Geometry: final body of the model. Coordinates: model frame, mm. A direction names the side the tool comes from. Give positions to 0.01 mm unless a question says otherwise; leave off trailing zeros. Write each loop counter-clockwise with the first axis right and the second up, starting at its lowest first coordinate (ties: lowest second). Pieces come first, ordered by that corner, then holes. Notation, with made-up numbers: M 47.25,86.25 L 96.25,86.25 A5 ccw 96.25,92.25 Z; hole C 36.5,42 d8. An arc over 180 degrees is marked long. Use one line per item in the form item = value. Start each with the question number.
Item 1: Section query D-D on x = -6.5. Return loops of the section in (y, z), then the cut area to 3 significant figures.
Item 2: Section query C-C on y = 0.5. Return loops of the section in (x, z), then the cut area to 3 significant figures.
Item 3: Section query A-A on x = -5. Return loops of the section in (y, z), then the cut area to 3 significant figures.
Item 4: Pull-direction query (Z, two-part tool) for faces 1 (the flat face through (-2, 1, -2.3)), 2 (the flat face through (0, 3, 0)), 3 (the flat face through (-2, 2, 2.8)), 4 (the flat face through (-4.15, 1, 1)); classes: released by +Z, released by -Z, zero draft, split by the parting line, or undercut.
Item 5: Contact query for flat-ended pins moving along their axis: P1, Ø3, axis at y = 2, z = -0.5, coming from the -X side; P2, Ø0.9, axis at y = 0.5, z = 2, coming from the -X side; P3, Ø2, axis at y = 4.5, z = -0.5, coming from the -X side. Output: stop coordinate, or through.
Item 6: Section query B-B on z = -0.8. Return loops of the section in (x, y).
Item 7: Access query for faces 5 (the flat face through (-5.5, 1, 2)), 6 (the flat face through (-5, 1, 1.65)), 7 (the flat face through (-3, 0, 0)). Directions: +Z, -Z, +X, -X, +Y, -Y. A direction counts if a zero-diameter tool reaches every point of the face in a straight line with its end or side. Return the directions, or none.
Item 8: Material intervals for line 1 along X through (y, z) = (1, 2.3); line 2 along X through (y, z) = (1.8, 0.2); line 3 along Y through (x, z) = (-4.5, 2.05), sorted ascending. Write a range as from..to.
from build123d import *

# Parameters (mm, degrees)
F1_DEPTH      = 2.3
F1_DEPTH_BACK = 2.8
F2_DEPTH      = 2.3
F3_DEPTH      = 1.65


with BuildPart() as f1:
    # F0 (on Top) → F1 (new body, two sides)
    with BuildSketch(Plane.XY) as f1_sk:
        Polygon((-4.15, 0), (0, 0), (0, 5.1), (-4.15, 2.55), align=None)
        Polygon((-5.5, 0), (-4.15, 0), (-4.15, 2.55), (-5.5, 1.7204819277), align=None)
    extrude(amount=-F1_DEPTH)
    extrude(f1_sk.sketch, amount=F1_DEPTH_BACK)

    # F0 (on Top) → F2 (join)
    with BuildSketch(Plane.XY):
        Polygon((-8.3, 0), (-5.5, 0), (-5.5, 1.7204819277), align=None)
    extrude(amount=-F2_DEPTH)

    # F0 (on Top) → F3 (cut)
    with BuildSketch(Plane.XY):
        Polygon((-5.5, 0), (-4.15, 0), (-4.15, 2.55), (-5.5, 1.7204819277), align=None)
    extrude(amount=F3_DEPTH, mode=Mode.SUBTRACT)


solid = f1.part
Answer sheet:
q1.outline = M 0,-2.3 L 1.11,-2.3 L 1.11,0 L 0,0 Z
q1.area = 2.54 mm2
q2.outline = M -7.49,-2.3 L 0,-2.3 L 0,2.8 L -5.5,2.8 L -5.5,1.65 L -4.15,1.65 L -4.15,0 L -7.49,0 Z
q2.area = 30.4 mm2
q3.outline = M 0,-2.3 L 2.03,-2.3 L 2.03,0 L 0,0 Z; M 0,1.65 L 2.03,1.65 L 2.03,2.8 L 0,2.8 Z
q3.area = 7.00 mm2
q4.face_1 = released by -Z
q4.face_2 = zero draft
q4.face_3 = released by +Z
q4.face_4 = undercut
q5.P1 = -7.49
q5.P2 = -5.5
q5.P3 = -2.6
q6.outline = M -8.3,0 L 0,0 L 0,5.1 Z
q7.face_5 = +Z, -X, +Y, -Y
q7.face_6 = -X, +Y, -Y
q7.face_7 = +Z, -Z, +X, -X, -Y
q8.line_1 = -5.5..0
q8.line_2 = -4.15..0
q8.line_3 = 0..2.33
